from build123d import *

# Parameters (mm, degrees)
SKETCH1_W           = 107
SKETCH1_H           = 57
SKETCH1_R           = 1.5
BOSS_EXTRUDE1_DEPTH = 3.175
FILLET1_R           = 2
CUT_EXTRUDE1_DEPTH  = 3.175


with BuildPart() as part:
    # Sketch1 → Boss-Extrude1 (new body)
    with BuildSketch(Plane.XY):
        Rectangle(SKETCH1_W, SKETCH1_H)
        with Locations((-50, 25)):
            Circle(SKETCH1_R, mode=Mode.SUBTRACT)
        with Locations((50, 25)):
            Circle(SKETCH1_R, mode=Mode.SUBTRACT)
        with Locations((-50, -25)):
            Circle(SKETCH1_R, mode=Mode.SUBTRACT)
        with Locations((50, -25)):
            Circle(SKETCH1_R, mode=Mode.SUBTRACT)
    extrude(amount=BOSS_EXTRUDE1_DEPTH)

    # Fillet1
    fillet1_edges = [part.edges().sort_by_distance(p)[0] for p in [
        (-53.5, 28.5, 1.5875),
        (53.5, 28.5, 1.5875),
        (53.5, -28.5, 1.5875),
        (-53.5, -28.5, 1.5875),
    ]]
    fillet(fillet1_edges, radius=FILLET1_R)

    # Sketch2 → Cut-Extrude1 (cut)
    with BuildSketch(Plane.XY.offset(3.175)):
        with BuildLine():
            Line((44.332340651, -7.787162566), (44.332340651, 7.787162566))
            ThreePointArc((44.332340651, 7.787162566), (47.5, 10.954821915), (50.667659349, 7.787162566))
            Line((50.667659349, 7.787162566), (50.667659349, -7.787162566))
            ThreePointArc((50.667659349, -7.787162566), (47.5, -10.954821915), (44.332340651, -7.787162566))
        make_face()
        with BuildLine():
            Line((-50.667659349, -7.787162566), (-50.667659349, 7.787162566))
            ThreePointArc((-50.667659349, 7.787162566), (-47.5, 10.954821915), (-44.332340651, 7.787162566))
            Line((-44.332340651, 7.787162566), (-44.332340651, -7.787162566))
            ThreePointArc((-44.332340651, -7.787162566), (-47.5, -10.954821915), (-50.667659349, -7.787162566))
        make_face()
        Polygon((14.43375673, 0), (7.216878365, 12.5), (-7.216878365, 12.5), (-14.43375673, 0), (-7.216878365, -12.5), (7.216878365, -12.5), align=None)
    extrude(amount=-CUT_EXTRUDE1_DEPTH, mode=Mode.SUBTRACT)


solid = part.part
Can you work these out from the model? Positions are in its coordinate system, mm. A direction names the side the tool comes from. Coordinates: 2 decimals unless noted, no trailing zeros. Order: outer loops, then holes, each group sorted by start corner. A loop starts at its lowest first (then second) coordinate and runs counter-clockwise, first axis right, second up. Notation, with made-up numbers: (65.5, -8) -> (101.5, -8) arc R12 cw to (101.5, 5) -> close; hole circle Ø10 at (53, 35.5). An arc over 180 degrees is marked (long way). Use one line per item in the form item = value.
Q1. We'd pull the mould along Y, two halves only. Please class faces 1 (the face through (52.9, -27.93, 1.61)), 2 (the face through (47.43, 10.954, 1.61)), 3 (the face through (52.9, 27.93, 1.61)): released by +Y, released by -Y, zero draft, split by the parting line, or undercut.
From the geometry:
face_1 = released by -Y
face_2 = undercut
face_3 = released by +Y
Q2. I need wall thicknesses on L1, parallel to X at y = -2.5, z = 1.65; L2, parallel to Y at x = -50, z = 1.55; L3, parallel to X at y = -1.5, z = 1.75. Which ranges of each line are inside material? Lowest first, please.
From the geometry:
L1 = -53.5 to -50.67, -44.33 to -12.99, 12.99 to 44.33, 50.67 to 53.5
L2 = -28.5 to -26.5, -23.5 to -9.73, 9.73 to 23.5, 26.5 to 28.5
L3 = -53.5 to -50.67, -44.33 to -13.57, 13.57 to 44.33, 50.67 to 53.5
Q3. Imagine slicing it at D-D, the plane x = -47.5. List the corners of the cut face in (y, z) for me (3 decimals).
From the geometry:
outline = (-28.5, 0) -> (-10.955, 0) -> (-10.955, 3.175) -> (-28.5, 3.175) -> close; (10.955, 0) -> (28.5, 0) -> (28.5, 3.175) -> (10.955, 3.175) -> close
Q4. Which directions (+Z, -Z, +X, -X, +Y, -Y) give clear straight access to the entire face, cutting with the end or side of a thin tool? Please do faces 4 (the face through (10.876, 6.163, 1.61)), 5 (the face through (-1, 28.5, 2)).
From the geometry:
face_4 = +Z, -Z
face_5 = +Z, -Z, +X, -X, +Y
Q5. Imagine slicing it at B-B, the plane y = -25. List the corners of the cut face in (x, z) for me (3 decimals).
From the geometry:
outline = (-53.5, 0) -> (-51.5, 0) -> (-51.5, 3.175) -> (-53.5, 3.175) -> close; (-48.5, 0) -> (48.5, 0) -> (48.5, 3.175) -> (-48.5, 3.175) -> close; (51.5, 0) -> (53.5, 0) -> (53.5, 3.175) -> (51.5, 3.175) -> close
Q6. Imagine slicing it at A-A, the plane z = 1.1. List the corners of the cut face in (x, y) for me.
From the geometry:
outline = (-53.5, -26.5) arc R2 ccw to (-51.5, -28.5) -> (51.5, -28.5) arc R2 ccw to (53.5, -26.5) -> (53.5, 26.5) arc R2 ccw to (51.5, 28.5) -> (-51.5, 28.5) arc R2 ccw to (-53.5, 26.5) -> close; hole circle Ø3 at (-50, -25); hole circle Ø3 at (-50, 25); hole (-50.67, -7.79) arc R3.17 ccw to (-44.33, -7.79) -> (-44.33, 7.79) arc R3.17 ccw to (-50.67, 7.79) -> close; hole (-14.43, 0) -> (-7.22, -12.5) -> (7.22, -12.5) -> (14.43, 0) -> (7.22, 12.5) -> (-7.22, 12.5) -> close; hole (44.33, -7.79) arc R3.17 ccw to (50.67, -7.79) -> (50.67, 7.79) arc R3.17 ccw to (44.33, 7.79) -> close; hole circle Ø3 at (50, -25); hole circle Ø3 at (50, 25)
Q7. Imagine slicing it at C-C, the plane x = 11.5. List the corners of the cut face in (y, z) for me (3 decimals).
From the geometry:
outline = (-28.5, 0) -> (-5.081, 0) -> (-5.081, 3.175) -> (-28.5, 3.175) -> close; (5.081, 0) -> (28.5, 0) -> (28.5, 3.175) -> (5.081, 3.175) -> close
